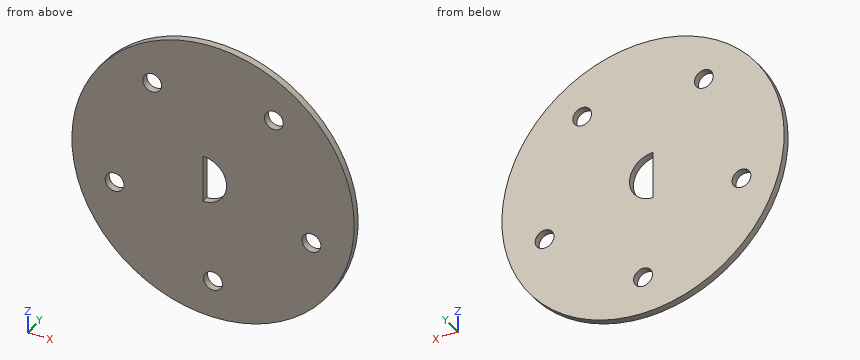
```python
from build123d import *

# Parameters (mm, degrees)
SKETCH1_R           = 38.1
SKETCH1_R_2         = 2.54
BOSS_EXTRUDE1_DEPTH = 1.89738


with BuildPart() as part:
    # Sketch1 → Boss-Extrude1 (new body)
    with BuildSketch(Plane(origin=(0, 0, 0), x_dir=(1, 0, 0), z_dir=(0, 1, 0))):
        with Locations(Location((0, 0, 0), (0, 0, 90))):
            Circle(SKETCH1_R)
        with Locations(Location((0, 27.94, 0), (0, 0, 90))):
            Circle(SKETCH1_R_2, mode=Mode.SUBTRACT)
        with Locations(Location((26.572519065, 8.633934823, 0), (0, 0, 90))):
            Circle(SKETCH1_R_2, mode=Mode.SUBTRACT)
        with Locations(Location((16.422719949, -22.603934823, 0), (0, 0, 90))):
            Circle(SKETCH1_R_2, mode=Mode.SUBTRACT)
        with Locations(Location((-16.422719949, -22.603934823, 0), (0, 0, 90))):
            Circle(SKETCH1_R_2, mode=Mode.SUBTRACT)
        with Locations(Location((-26.572519065, 8.633934823, 0), (0, 0, 90))):
            Circle(SKETCH1_R_2, mode=Mode.SUBTRACT)
        with BuildLine():
            Line((-2.695023706, 6.35), (-2.695023706, -6.35))
            ThreePointArc((-2.695023706, -6.35), (3.654976294, 0), (-2.695023706, 6.35))
        make_face(mode=Mode.SUBTRACT)
    extrude(amount=BOSS_EXTRUDE1_DEPTH)


solid = part.part
```
Build history of the part. All positions in model axes, mm. Round coordinates to 2 decimals unless told otherwise and drop trailing zeros. Loops run counter-clockwise (first coordinate to the right, second up) from the corner with the lowest first, then second, coordinate; pieces in that order, holes last.
Item 1: Saw through at B-B (x = 0). List the corners of the cut face in (y, z).
Item 2: Pin check, flat tips, straight feed: P1, Ø4, axis at x = 0, z = -27.94, coming from the +Y side; P2, Ø6.5, axis at x = -16.42, z = 22.6, coming from the -Y side; P3, Ø0.9, axis at y = 0.5, z = -1.5, coming from the +X side. Stop position of each tip, or through.
Item 3: Saw through at D-D (z = -27.94). List the corners of the cut face in (x, y).
Item 4: Saw through at C-C (y = 0.4). List the corners of the cut face in (x, z), then the cut area to 3 significant figures.
Item 5: Saw through at A-A (z = 0). List the corners of the cut face in (x, y).
Item 6: Drill centre lines: line 1 along X through (y, z) = (0.75, -10); line 2 along X through (y, z) = (1.35, 21.5); line 3 along X through (y, z) = (0.55, -27.94). Where is each one in solid material? Low to high.
Worked answers:
1. outline: (0, -38.1) - (1.9, -38.1) - (1.9, -30.48) - (0, -30.48) - close; (0, -25.4) - (1.9, -25.4) - (1.9, -5.75) - (0, -5.75) - close; (0, 5.75) - (1.9, 5.75) - (1.9, 38.1) - (0, 38.1) - close
2. P1: passes through
2. P2: stops at y = 0
2. P3: stops at x = 38.09
3. outline: (-25.9, 0) - (-2.54, 0) - (-2.54, 1.9) - (-25.9, 1.9) - close; (2.54, 0) - (25.9, 0) - (25.9, 1.9) - (2.54, 1.9) - close
4. outline: circle Ø76.2 at (0, 0); hole circle Ø5.08 at (-26.57, -8.63); hole circle Ø5.08 at (-16.42, 22.6); hole (-2.7, -6.35) arc R6.35 ccw to (-2.7, 6.35) - close; hole circle Ø5.08 at (0, -27.94); hole circle Ø5.08 at (16.42, 22.6); hole circle Ø5.08 at (26.57, -8.63)
4. area: 4,400 mm2
5. outline: (-38.1, 0) - (-2.7, 0) - (-2.7, 1.9) - (-38.1, 1.9) - close; (3.65, 0) - (38.1, 0) - (38.1, 1.9) - (3.65, 1.9) - close
6. line 1: x = -36.76 to -28.71, -24.43 to 24.43, 28.71 to 36.76
6. line 2: x = -31.45 to -18.71, -14.14 to 14.14, 18.71 to 31.45
6. line 3: x = -25.9 to -2.54, 2.54 to 25.9
